Design review of the part built by this model. Coordinates are the model's own, in mm. Round coordinates to 2 decimals unless told otherwise and drop trailing zeros. Use a Markdown table: item, result.
from build123d import *

# Parameters (mm, degrees)
F1_DEPTH = 228.6
F2_R     = 25.4


with BuildPart() as f1:
    # F0 (on Right) → F1 (new body, symmetric)
    with BuildSketch(Plane.YZ):
        with BuildLine():
            ThreePointArc((-397.279083, 225.959099), (-461.086876, 183.29803), (-410.897082, 125.225783))
            Line((-410.897082, 125.225783), (-46.446397, 14.155093))
            ThreePointArc((-46.446397, 14.155093), (31.406704, 51.789828), (0, 132.357175))
            ThreePointArc((0, 132.357175), (-45.230298, 141.1617), (-88.834917, 126.264159))
            ThreePointArc((-88.834917, 126.264159), (-136.030627, 124.157236), (-183.226337, 126.264159))
            ThreePointArc((-183.226337, 126.264159), (-295.26164, 165.357068), (-397.279083, 225.959099))
        make_face()
    extrude(amount=F1_DEPTH, both=True)

    # F2
    f2_edges = [f1.edges().sort_by_distance(p)[0] for p in [
        (-228.6, -461.086876, 183.29803),
        (-228.6, -228.671739, 69.690438),
        (-228.6, 31.406704, 51.789828),
        (-228.6, -45.230298, 141.1617),
        (-228.6, -136.030627, 124.157236),
        (-228.6, -295.26164, 165.357068),
        (228.6, -461.086876, 183.29803),
        (228.6, -228.671739, 69.690438),
        (228.6, 31.406704, 51.789828),
        (228.6, -45.230298, 141.1617),
        (228.6, -136.030627, 124.157236),
        (228.6, -295.26164, 165.357068),
        (0, -183.226337, 126.264159),
        (0, -88.834917, 126.264159),
        (0, 0, 132.357175),
        (0, -397.279083, 225.959099),
        (0, -410.897082, 125.225783),
        (0, -46.446397, 14.155093),
    ]]
    fillet(f2_edges, radius=F2_R)


solid = f1.part
1. Wall thickness on line 1 along Z through (x, y) = (-17.5, 0.5); line 2 along Z through (x, y) = (123.5, -360); line 3 along Y through (x, z) = (-17, 181.5): over which ranges is each line inside the solid? List them lowest first. Write a range as from..to.
Check values:
| item | result |
|---|---|
| line 1 | z = 18.06..132.11 |
| line 2 | z = 109.71..200.56 |
| line 3 | y = -461.3..-327.35 |
2. Insertion check: pin 1 (10 mm diameter, centred on x = -25.5, y = -318.5, fed in from -Z); pin 2 (4 mm diameter, centred on x = -166.5, z = 187.5, fed in from +Y); pin 3 (12 mm diameter, centred on x = -59, y = -206, fed in from +Z). Each pin has a flat end and moves straight along its axis. Give the tip position at first contact, or say it passes through.
Check values:
| item | result |
|---|---|
| pin 1 | stops at z = 95.54 |
| pin 2 | stops at y = -334.61 |
| pin 3 | stops at z = 133.94 |
3. The part is to be moulded in two halves that separate along Y. For faces 1 (the face through (2.84, -137.6, 124.16)), 2 (the face through (228.6, -181, 95)), 3 (the face through (2.84, -292.17, 163.93)), 4 (the face through (221.36, -222.35, 75.75)), say which applies: pulls with the +Y half, pulls with the -Y half, needs draft (parallel to the pull), parting line crosses it, or undercut.
Check values:
| item | result |
|---|---|
| face 1 | undercut |
| face 2 | needs draft |
| face 3 | undercut |
| face 4 | pulls with the -Y half |
